from build123d import *

# Parameters (mm, degrees)
F0_W        = 228.6
F0_H        = 50
F1_DEPTH    = 50
F3_DEPTH    = 48
F4_R        = 11
F5_DEPTH    = 9
F7_DEPTH    = 15
F8_T2_ANGLE = 343.7894292622


# Not quite as in the source:
# - a fillet or chamfer that OpenCascade refuses, or shapes differently, is made with other operations: its cross-section is extruded or revolved along the edge and cut away or added


with BuildPart() as f1:
    # F0 (on Front) → F1 (new body)
    with BuildSketch(Plane.XZ):
        Rectangle(F0_W, F0_H)
    extrude(amount=F1_DEPTH)

    # F2 (on face) → F3 (cut)
    with BuildSketch(Plane(origin=(0, 0, 0), x_dir=(-1, 0, 0), z_dir=(0, 1, 0))):
        Polygon((-106.0638769388, 21.0001030612), (-110.06398, 17), (-110.06398, -17), (-106.0638769388, -21.0001030612), (-72.0638769388, -21.0001030612), (-68.0637738777, -17), (-68.0637738777, 17), (-72.0638769388, 21.0001030612), align=None)
    extrude(amount=-F3_DEPTH, mode=Mode.SUBTRACT)

    # F4 (on face) → F5 (cut)
    with BuildSketch(Plane(origin=(0, 0, 0), x_dir=(-1, 0, 0), z_dir=(0, 1, 0))):
        with Locations((89.3, 0)):
            Circle(F4_R)
    extrude(amount=-F5_DEPTH, mode=Mode.SUBTRACT)

    # F6 (on face) → F7 (cut)
    with BuildSketch(Plane(origin=(0, -9, 0), x_dir=(-1, 0, 0), z_dir=(0, 1, 0))):
        with BuildLine():
            Line((90.8, 2), (87.8, 2))
            ThreePointArc((87.8, 2), (89.3, -2.5), (90.8, 2))
        make_face()
    extrude(amount=-F7_DEPTH, mode=Mode.SUBTRACT)

    # F8: fillet of radius 0.5 on 1 edges, made by hand

    # F8_s1 → F8_t2 (revolve)
    with BuildSketch(Plane(origin=(-87.5248141005, 0, 12.4648632504), x_dir=(0, 1, 0), z_dir=(-0.9900106558, 0, 0.1409925581))):
        with BuildLine():
            ThreePointArc((-23.5, 10.0906354418), (-23.8535533906, 10.2370820512), (-24, 10.5906354418))
            Line((-24, 10.5906354418), (-24, 10.0906354418))
            Line((-24, 10.0906354418), (-23.5, 10.0906354418))
        make_face()
    revolve(axis=Axis((-89.3, -24, 0), (0, 1, 0)), revolution_arc=F8_T2_ANGLE)


solid = f1.part
Source: CAD feature listing. Evaluate the final solid. Frame: model axes, mm. A direction names the side the tool comes from. Give positions to 0.01 mm unless a question says otherwise; leave off trailing zeros. Order: outer loops, then holes, each group sorted by start corner. A loop starts at its lowest first (then second) coordinate and runs counter-clockwise, first axis right, second up. Notation, with made-up numbers: (72, -37) -> (89, -37) arc R17 cw to (89, -25) -> close; hole circle Ø7 at (-25, -35.5). An arc over 180 degrees is marked (long way). Write item = value, one per line.
Item 1: Section query C-C (z = 0). Output: boundary loops of the cut face in (x, y).
Check result:
outline = (-114.3, -50) -> (114.3, -50) -> (114.3, 0) -> (110.06, 0) -> (110.06, -48) -> (68.06, -48) -> (68.06, 0) -> (-78.3, 0) -> (-78.3, -9) -> (-86.8, -9) -> (-86.8, -23.5) arc R0.5 cw to (-87.3, -24) -> (-91.3, -24) arc R0.5 cw to (-91.8, -23.5) -> (-91.8, -9) -> (-100.3, -9) -> (-100.3, 0) -> (-114.3, 0) -> close
Item 2: Section query D-D (x = -81.5). Output: boundary loops of the cut face in (y, z).
Check result:
outline = (-50, -25) -> (0, -25) -> (0, -7.76) -> (-9, -7.76) -> (-9, 7.76) -> (0, 7.76) -> (0, 25) -> (-50, 25) -> close
Item 3: Section query A-A (y = -39.5). Output: boundary loops of the cut face in (x, z), then the cut area to 3 significant figures.
Check result:
outline = (-114.3, -25) -> (114.3, -25) -> (114.3, 25) -> (-114.3, 25) -> close; hole (68.06, -17) -> (72.06, -21) -> (106.06, -21) -> (110.06, -17) -> (110.06, 17) -> (106.06, 21) -> (72.06, 21) -> (68.06, 17) -> close
area = 9,700 mm²
Item 4: Mould query, pull axis Z, two halves, no side actions, for faces 1 (the face through (-89, -24, 0)), 2 (the face through (-2, -50, 0)), 3 (the face through (-2, -25, -25)). Classes: +Z half, -Z half, draft (parallel to the pull), parting line (faces both ways), or undercut.
Check result:
face_1 = undercut
face_2 = draft
face_3 = -Z half
Item 5: Set-up query: faces 4 (the face through (-27, 0, 0)), 5 (the face through (-86.92, -4.44, -10.74)). Return all of +Z, -Z, +X, -X, +Y, -Y with unobstructed straight access to the full face (end or side cutting, diameter ignored); none if empty.
Check result:
face_4 = +Z, -Z, +X, -X, +Y
face_5 = +Y
Item 6: Ray query, probe 1 along X at (y, z) = (-12.75, 0); probe 2 along Z at (x, y) = (-89.3, -12.75); probe 3 along X at (y, z) = (-28.5, 7). Return the intervals inside material, ascending.
Check result:
probe_1 = -114.3 to -91.8, -86.8 to 68.06, 110.06 to 114.3
probe_2 = -25 to -2.5, 2 to 25
probe_3 = -114.3 to 68.06, 110.06 to 114.3
Item 7: Section query B-B (y = -13.5). Output: boundary loops of the cut face in (x, z).
Check result:
outline = (-114.3, -25) -> (114.3, -25) -> (114.3, 25) -> (-114.3, 25) -> close; hole (-90.8, 2) arc R2.5 ccw (long way) to (-87.8, 2) -> close; hole (68.06, -17) -> (72.06, -21) -> (106.06, -21) -> (110.06, -17) -> (110.06, 17) -> (106.06, 21) -> (72.06, 21) -> (68.06, 17) -> close
Item 8: Contact query for flat-ended pins moving along their axis: pin 1 (13 mm diameter, centred on x = -89.3, z = 0, fed in from +Y); pin 2 (1.2 mm diameter, centred on x = -89, z = 1, fed in from +Y). Output: stop coordinate, or through.
Check result:
pin_1 = -9
pin_2 = -24
